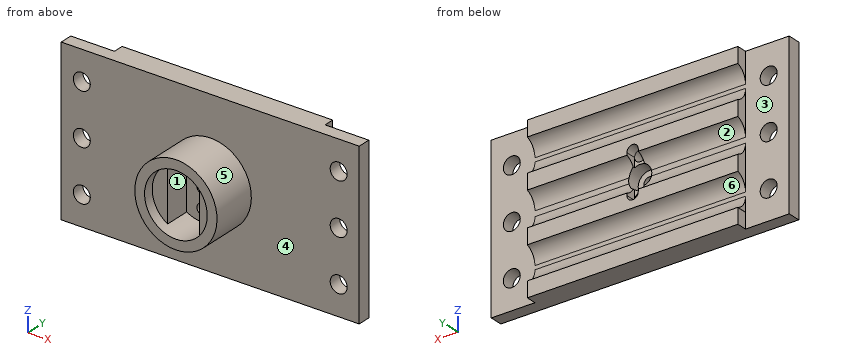
from build123d import *

# Parameters (mm, degrees)
SKETCH_1_R               = 50
EXTRUDE_1_DEPTH          = 2.5
SKETCH_2_R               = 8
EXTRUDE_2_DEPTH          = 9
SKETCH_3_R               = 6.1
CUT_EXTRUDE_1_DEPTH      = 2
CUT_EXTRUDE_2_DEPTH      = 5
SKETCH_7_R               = 1.15
CUT_EXTRUDE_4_DEPTH      = 4.5
SKETCH_8_R               = 2.25
CUT_EXTRUDE_5_DEPTH      = 2.5
CUT_EXTRUDE_6_DEPTH      = 72.281133549
CUT_EXTRUDE_6_DEPTH_BACK = 72.281133549
SKETCH_11_R              = 1.1
SKETCH_14_R              = 1.65
CUT_EXTRUDE_7_DEPTH      = 2.5
CUT_EXTRUDE_START        = -2.5
SKETCH_15_R              = 50
SKETCH_15_W              = 58
SKETCH_15_H              = 31.5
CUT_EXTRUDE_8_DEPTH      = 2.5
SKETCH_16_W              = 41
SKETCH_16_H              = 3
EXTRUDE_4_DEPTH          = 2
CUT_EXTRUDE_9_DEPTH      = 2
FILLET_3_R               = 3


with BuildPart() as part:
    # Эскиз1 → Бобышка-Вытянуть1 (new body)
    with BuildSketch(Plane(origin=(0, 0, 0), x_dir=(1, 0, 0), z_dir=(0, 1, 0))):
        with Locations(Location((0, 0, 0), (0, 0, 270))):
            Circle(SKETCH_1_R)
    extrude(amount=EXTRUDE_1_DEPTH)

    # Эскиз2 → Бобышка-Вытянуть2 (add)
    with BuildSketch(Plane.XZ):
        with Locations(Location((0, 0, 0), (0, 0, 270))):
            Circle(SKETCH_2_R)
    extrude(amount=EXTRUDE_2_DEPTH)

    # Эскиз3 → Вырез-Вытянуть1 (cut)
    with BuildSketch(Plane.XZ.offset(9)):
        with Locations(Location((0, 0, 0), (0, 0, 270))):
            Circle(SKETCH_3_R)
    extrude(amount=-CUT_EXTRUDE_1_DEPTH, mode=Mode.SUBTRACT)

    # Эскиз4 → Вырез-Вытянуть2 (cut)
    with BuildSketch(Plane.XZ.offset(7)):
        with BuildLine():
            Line((-3.1, 5.253570215), (-3.1, -5.253570215))
            ThreePointArc((-3.1, -5.253570215), (0, -6.1), (3.1, -5.253570215))
            Line((3.1, -5.253570215), (3.1, 5.253570215))
            ThreePointArc((3.1, 5.253570215), (0, 6.1), (-3.1, 5.253570215))
        make_face()
    extrude(amount=-CUT_EXTRUDE_2_DEPTH, mode=Mode.SUBTRACT)

    # Эскиз7 → Вырез-Вытянуть4 (cut)
    with BuildSketch(Plane(origin=(0, 2.5, 0), x_dir=(1, 0, 0), z_dir=(0, 1, 0))):
        with Locations(Location((0, 0, 0), (0, 0, 270))):
            Circle(SKETCH_7_R)
    extrude(amount=-CUT_EXTRUDE_4_DEPTH, mode=Mode.SUBTRACT)

    # Эскиз8 → Вырез-Вытянуть5 (cut)
    with BuildSketch(Plane(origin=(0, 2.5, 0), x_dir=(1, 0, 0), z_dir=(0, 1, 0))):
        with Locations(Location((0, 0, 0), (0, 0, 270))):
            Circle(SKETCH_8_R)
    extrude(amount=-CUT_EXTRUDE_5_DEPTH, mode=Mode.SUBTRACT)

    # Эскиз11 → Вырез-Вытянуть6 (cut, two sides: drawn at the far end of the back side and taken through both)
    with BuildSketch(Plane.XZ.offset(-CUT_EXTRUDE_6_DEPTH_BACK)):
        with Locations(Location((0, 3.8, 0), (0, 0, 270))):
            Circle(SKETCH_11_R)
        with Locations(Location((0, -3.8, 0), (0, 0, 90))):
            Circle(SKETCH_11_R)
    extrude(amount=CUT_EXTRUDE_6_DEPTH + CUT_EXTRUDE_6_DEPTH_BACK, mode=Mode.SUBTRACT)

    # Эскиз14 → Вырез-Вытянуть7 (cut)
    with BuildSketch(Plane(origin=(0, 2.5, 0), x_dir=(1, 0, 0), z_dir=(0, 1, 0))):
        with Locations(Location((-25, 0, 0), (0, 0, 270))):
            Circle(SKETCH_14_R)
        with Locations(Location((-25, 10, 0), (0, 0, 270))):
            Circle(SKETCH_14_R)
        with Locations(Location((-25, -10, 0), (0, 0, 270))):
            Circle(SKETCH_14_R)
        with Locations(Location((25, -10, 0), (0, 0, 270))):
            Circle(SKETCH_14_R)
        with Locations(Location((25, 0, 0), (0, 0, 270))):
            Circle(SKETCH_14_R)
        with Locations(Location((25, 10, 0), (0, 0, 270))):
            Circle(SKETCH_14_R)
    extrude(amount=-CUT_EXTRUDE_7_DEPTH, mode=Mode.SUBTRACT)

    # Эскиз15 → Вырез-Вытянуть8 (cut)
    with BuildSketch(Plane(origin=(0, 2.5, 0), x_dir=(1, 0, 0), z_dir=(0, 1, 0)).offset(CUT_EXTRUDE_START)):
        Circle(SKETCH_15_R)
        Rectangle(SKETCH_15_W, SKETCH_15_H, mode=Mode.SUBTRACT)
    extrude(amount=CUT_EXTRUDE_8_DEPTH, mode=Mode.SUBTRACT)

    # Эскиз16 → Бобышка-Вытянуть4 (add)
    with BuildSketch(Plane(origin=(0, 2.5, 0), x_dir=(1, 0, 0), z_dir=(0, 1, 0))):
        with Locations((0, 14.25)):
            Rectangle(SKETCH_16_W, SKETCH_16_H)
        with Locations((0, 4.85)):
            Rectangle(SKETCH_16_W, SKETCH_16_H)
        with Locations((0, -4.85)):
            Rectangle(SKETCH_16_W, SKETCH_16_H)
        with Locations((0, -14.25)):
            Rectangle(SKETCH_16_W, SKETCH_16_H)
    extrude(amount=EXTRUDE_4_DEPTH)

    # Эскиз17 → Вырез-Вытянуть9 (cut)
    with BuildSketch(Plane(origin=(0, 2.5, 0), x_dir=(1, 0, 0), z_dir=(0, 1, 0))):
        with BuildLine():
            Line((-1.1, 3.8), (-1.1, 2.7))
            Line((-1.1, 2.7), (1.1, 2.7))
            Line((1.1, 2.7), (1.1, 3.8))
            ThreePointArc((1.1, 3.8), (0, 4.9), (-1.1, 3.8))
        make_face()
        with BuildLine():
            Line((-1.1, -3.8), (-1.1, -2.7))
            Line((-1.1, -2.7), (1.1, -2.7))
            Line((1.1, -2.7), (1.1, -3.8))
            ThreePointArc((1.1, -3.8), (0, -4.9), (-1.1, -3.8))
        make_face()
    extrude(amount=CUT_EXTRUDE_9_DEPTH, mode=Mode.SUBTRACT)

    # Скругление3
    # the kernel refuses this fillet: 3 mm, written as the material it adds along each edge
    with BuildSketch(Plane(origin=(20.5, 2.5, 12.75), x_dir=(0, 0, -1), z_dir=(-1, 0, 0)), Plane(origin=(-20.5, 2.5, 6.35), x_dir=(0, 0, 1), z_dir=(1, 0, 0))) as fillet_3_piece_1:
        with BuildLine():
            CenterArc((2.828427125, -3), FILLET_3_R, 90, 70.528779366)
            Line((0, -2), (-0.056568542, -1.98))
            ThreePointArc((-0.056568542, -1.98), (-0.06, -1), (-0.06, 0))
            Line((-0.06, 0), (0, 0.06))
            Line((0, 0.06), (2.828427125, 0.06))
            Line((2.828427125, 0.06), (2.828427125, 0))
        make_face()
    extrude(amount=41)
    with BuildSketch(Plane(origin=(20.5, 2.5, 3.35), x_dir=(0, 0, -1), z_dir=(-1, 0, 0))) as fillet_3_piece_2_section:
        with BuildLine():
            CenterArc((2.828427125, -3), FILLET_3_R, 90, 70.528779366)
            Line((0, -2), (-0.056568542, -1.98))
            ThreePointArc((-0.056568542, -1.98), (-0.06, -1), (-0.06, 0))
            Line((-0.06, 0), (0, 0.06))
            Line((0, 0.06), (2.828427125, 0.06))
            Line((2.828427125, 0.06), (2.828427125, 0))
        make_face()
    fillet_3_piece_2 = extrude(amount=19.4, mode=Mode.PRIVATE)
    fillet_3_piece_2 = fillet_3_piece_2 - Plane(origin=(0, 3.015381172, 0), x_dir=(0, 0, 1), z_dir=(0, 1, 0)) * Cylinder(2.25, 51, mode=Mode.PRIVATE)
    add(fillet_3_piece_2)
    with BuildSketch(Plane(origin=(20.5, 2.5, 3.35), x_dir=(0, 0, -1), z_dir=(-1, 0, 0))) as fillet_3_piece_3_section:
        with BuildLine():
            CenterArc((2.828427125, -3), FILLET_3_R, 90, 70.528779366)
            Line((0, -2), (-0.056568542, -1.98))
            ThreePointArc((-0.056568542, -1.98), (-0.06, -1), (-0.06, 0))
            Line((-0.06, 0), (0, 0.06))
            Line((0, 0.06), (2.828427125, 0.06))
            Line((2.828427125, 0.06), (2.828427125, 0))
        make_face()
    fillet_3_piece_3 = extrude(amount=26.471067812, mode=Mode.PRIVATE)
    fillet_3_piece_3 = fillet_3_piece_3 - Plane(origin=(0, 3.020982336, 0), x_dir=(0, 0, 1), z_dir=(0, 1, 0)) * Cylinder(2.25, 65, mode=Mode.PRIVATE)
    fillet_3_piece_3 = split(fillet_3_piece_3, bisect_by=Plane(origin=(-1.1, 3.020982336, 2.69327095), z_dir=(-1, 0, 0)), keep=Keep.TOP, mode=Mode.PRIVATE)
    add(fillet_3_piece_3)
    with BuildSketch(Plane(origin=(5.971067812, 2.5, 3.35), x_dir=(0, 0, -1), z_dir=(-1, 0, 0))) as fillet_3_piece_4_section:
        with BuildLine():
            CenterArc((2.828427125, -3), FILLET_3_R, 90, 70.528779366)
            Line((0, -2), (-0.056568542, -1.98))
            ThreePointArc((-0.056568542, -1.98), (-0.06, -1), (-0.06, 0))
            Line((-0.06, 0), (0, 0.06))
            Line((0, 0.06), (2.828427125, 0.06))
            Line((2.828427125, 0.06), (2.828427125, 0))
        make_face()
    fillet_3_piece_4 = extrude(amount=26.471067812, mode=Mode.PRIVATE)
    fillet_3_piece_4 = fillet_3_piece_4 - Plane(origin=(0, 3.020982326, 0), x_dir=(0, 0, 1), z_dir=(0, 1, 0)) * Cylinder(2.25, 65, mode=Mode.PRIVATE)
    fillet_3_piece_4 = split(fillet_3_piece_4, bisect_by=Plane(origin=(1.1, 3.020982326, 2.69327092), z_dir=(1, 0, 0)), keep=Keep.TOP, mode=Mode.PRIVATE)
    add(fillet_3_piece_4)
    with BuildSketch(Plane(origin=(-1.1, 2.5, 3.35), x_dir=(0, 0, -1), z_dir=(-1, 0, 0))) as fillet_3_piece_5_section:
        with BuildLine():
            CenterArc((2.828427125, -3), FILLET_3_R, 90, 70.528779366)
            Line((0, -2), (-0.056568542, -1.98))
            ThreePointArc((-0.056568542, -1.98), (-0.06, -1), (-0.06, 0))
            Line((-0.06, 0), (0, 0.06))
            Line((0, 0.06), (2.828427125, 0.06))
            Line((2.828427125, 0.06), (2.828427125, 0))
        make_face()
    fillet_3_piece_5 = extrude(amount=19.4, mode=Mode.PRIVATE)
    fillet_3_piece_5 = fillet_3_piece_5 - Plane(origin=(0, 3.015381179, 0), x_dir=(0, 0, 1), z_dir=(0, 1, 0)) * Cylinder(2.25, 51, mode=Mode.PRIVATE)
    add(fillet_3_piece_5)
    with BuildSketch(Plane(origin=(5.971067812, 2.5, -3.35), x_dir=(0, 0, 1), z_dir=(-1, 0, 0))) as fillet_3_piece_6_section:
        with BuildLine():
            CenterArc((2.828427125, 3), FILLET_3_R, 199.471220634, 70.528779366)
            Line((0, 2), (-0.056568542, 1.98))
            ThreePointArc((-0.056568542, 1.98), (-0.06, 1), (-0.06, 0))
            Line((-0.06, 0), (0, -0.06))
            Line((0, -0.06), (2.828427125, -0.06))
            Line((2.828427125, -0.06), (2.828427125, 0))
        make_face()
    fillet_3_piece_6 = extrude(amount=26.471067812, mode=Mode.PRIVATE)
    fillet_3_piece_6 = fillet_3_piece_6 - Plane(origin=(0, 3.020982336, 0), x_dir=(0, 0, 1), z_dir=(0, 1, 0)) * Cylinder(2.25, 65, mode=Mode.PRIVATE)
    fillet_3_piece_6 = split(fillet_3_piece_6, bisect_by=Plane(origin=(1.1, 3.020982336, -2.69327095), z_dir=(1, 0, 0)), keep=Keep.TOP, mode=Mode.PRIVATE)
    add(fillet_3_piece_6)
    with BuildSketch(Plane(origin=(-1.1, 2.5, -3.35), x_dir=(0, 0, 1), z_dir=(-1, 0, 0))) as fillet_3_piece_7_section:
        with BuildLine():
            CenterArc((2.828427125, 3), FILLET_3_R, 199.471220634, 70.528779366)
            Line((0, 2), (-0.056568542, 1.98))
            ThreePointArc((-0.056568542, 1.98), (-0.06, 1), (-0.06, 0))
            Line((-0.06, 0), (0, -0.06))
            Line((0, -0.06), (2.828427125, -0.06))
            Line((2.828427125, -0.06), (2.828427125, 0))
        make_face()
    fillet_3_piece_7 = extrude(amount=19.4, mode=Mode.PRIVATE)
    fillet_3_piece_7 = fillet_3_piece_7 - Plane(origin=(0, 3.015381172, 0), x_dir=(0, 0, 1), z_dir=(0, 1, 0)) * Cylinder(2.25, 51, mode=Mode.PRIVATE)
    add(fillet_3_piece_7)
    with BuildSketch(Plane(origin=(20.5, 2.5, -3.35), x_dir=(0, 0, 1), z_dir=(-1, 0, 0))) as fillet_3_piece_8_section:
        with BuildLine():
            CenterArc((2.828427125, 3), FILLET_3_R, 199.471220634, 70.528779366)
            Line((0, 2), (-0.056568542, 1.98))
            ThreePointArc((-0.056568542, 1.98), (-0.06, 1), (-0.06, 0))
            Line((-0.06, 0), (0, -0.06))
            Line((0, -0.06), (2.828427125, -0.06))
            Line((2.828427125, -0.06), (2.828427125, 0))
        make_face()
    fillet_3_piece_8 = extrude(amount=19.4, mode=Mode.PRIVATE)
    fillet_3_piece_8 = fillet_3_piece_8 - Plane(origin=(0, 3.015381179, 0), x_dir=(0, 0, 1), z_dir=(0, 1, 0)) * Cylinder(2.25, 51, mode=Mode.PRIVATE)
    add(fillet_3_piece_8)
    with BuildSketch(Plane(origin=(20.5, 2.5, -3.35), x_dir=(0, 0, 1), z_dir=(-1, 0, 0))) as fillet_3_piece_9_section:
        with BuildLine():
            CenterArc((2.828427125, 3), FILLET_3_R, 199.471220634, 70.528779366)
            Line((0, 2), (-0.056568542, 1.98))
            ThreePointArc((-0.056568542, 1.98), (-0.06, 1), (-0.06, 0))
            Line((-0.06, 0), (0, -0.06))
            Line((0, -0.06), (2.828427125, -0.06))
            Line((2.828427125, -0.06), (2.828427125, 0))
        make_face()
    fillet_3_piece_9 = extrude(amount=26.471067812, mode=Mode.PRIVATE)
    fillet_3_piece_9 = fillet_3_piece_9 - Plane(origin=(0, 3.020982325, 0), x_dir=(0, 0, 1), z_dir=(0, 1, 0)) * Cylinder(2.25, 65, mode=Mode.PRIVATE)
    fillet_3_piece_9 = split(fillet_3_piece_9, bisect_by=Plane(origin=(-1.1, 3.020982325, -2.69327092), z_dir=(-1, 0, 0)), keep=Keep.TOP, mode=Mode.PRIVATE)
    add(fillet_3_piece_9)
    with BuildSketch(Plane(origin=(-20.5, 2.5, -6.35), x_dir=(0, 0, -1), z_dir=(1, 0, 0)), Plane(origin=(20.5, 2.5, -12.75), x_dir=(0, 0, 1), z_dir=(-1, 0, 0))) as fillet_3_piece_10:
        with BuildLine():
            CenterArc((2.828427125, 3), FILLET_3_R, 199.471220634, 70.528779366)
            Line((0, 2), (-0.056568542, 1.98))
            ThreePointArc((-0.056568542, 1.98), (-0.06, 1), (-0.06, 0))
            Line((-0.06, 0), (0, -0.06))
            Line((0, -0.06), (2.828427125, -0.06))
            Line((2.828427125, -0.06), (2.828427125, 0))
        make_face()
    extrude(amount=41)


solid = part.part
Read the model definition and answer for the solid it produces. Units are mm, in the model's axes. Face numbers are marked on the shaded views. A direction names the side the tool comes from. Give positions to 0.01 mm unless a question says otherwise; leave off trailing zeros. Write each loop counter-clockwise with the first axis right and the second up, starting at its lowest first coordinate (ties: lowest second). Pieces come first, ordered by that corner, then holes. Notation, with made-up numbers: (14, 47.25) - (30, 47.25) arc R15 ccw to (30, 52.25) - close; hole circle Ø3 at (57.5, 85.5). An arc over 180 degrees is marked (long way). Use CSV: the item, a comma, the result in double quotes. Start each with the question number.
Item 1: The part is cut by section B-B, the plane z = -11. Give the vertices of the cut face in (x, y).
Item 2: Consider line 1 (X direction, y = 1.5, z = 10); line 2 (X direction, y = 1.4, z = 0); line 3 (X direction, y = -5.25, z = 0). Determine where each line is inside the solid, lowest interval first.
Item 3: The part is cut by section A-A, the plane x = 25. Give the vertices of the cut face in (y, z).
Item 4: The part is cut by section D-D, the plane y = -1.25. Give the vertices of the cut face in (x, z), and give its area (3 significant figures).
Item 5: Flat-ended cylindrical pins translate along their axes: P1, Ø0.6, axis at y = 3.5, z = -5.5, coming from the -X side; P2, Ø5, axis at x = 0, z = 0.5, coming from the +Y side; P3, Ø3, axis at x = 0, z = -3.8, coming from the -Y side; P4, Ø8, axis at x = -17.5, y = -6.5, coming from the +Z side. Find the tip coordinate at first contact, or state that the pin passes through.
Item 6: The part is cut by section C-C, the plane y = -4.5. Give the vertices of the cut face in (x, z), and give its area (3 significant figures).
Item 7: The mould has two halves that part along Z. Classify the marked faces 4, 5 and 6: pulls with the +Z half, pulls with the -Z half, needs draft (parallel to the pull), parting line crosses it, or undercut.
Item 8: For the marked faces 1, 2 and 3, determine the directions among +Z, -Z, +X, -X, +Y, -Y from which every point of the face is accessible in a straight line to the end or side of a thin tool.
Taken from the geometry:
1,outline,"(-29, 0) - (-26.31, 0) - (-26.31, 2.5) - (-29, 2.5) - close; (-23.69, 0) - (23.69, 0) - (23.69, 2.5) - (20.5, 2.5) - (20.5, 2.7) - (-20.5, 2.7) - (-20.5, 2.5) - (-23.69, 2.5) - close; (26.31, 0) - (29, 0) - (29, 2.5) - (26.31, 2.5) - close"
2,line 1,"-29 to -26.65, -23.35 to 23.35, 26.65 to 29"
2,line 2,"-29 to -26.65, -23.35 to -2.25, 2.25 to 23.35, 26.65 to 29"
2,line 3,"-8 to -3.1, 3.1 to 8"
3,outline,"(0, -15.75) - (2.5, -15.75) - (2.5, -11.65) - (0, -11.65) - close; (0, -8.35) - (2.5, -8.35) - (2.5, -1.65) - (0, -1.65) - close; (0, 1.65) - (2.5, 1.65) - (2.5, 8.35) - (0, 8.35) - close; (0, 11.65) - (2.5, 11.65) - (2.5, 15.75) - (0, 15.75) - close"
4,outline,"circle Ø16 at (0, 0); hole circle Ø2.3 at (0, 0); hole circle Ø2.2 at (0, -3.8); hole circle Ø2.2 at (0, 3.8)"
4,area,"189 mm2"
5,P1,"x = -20.5"
5,P2,"y = 3.49"
5,P3,"y = -2"
5,P4,"through"
6,outline,"circle Ø16 at (0, 0); hole (-3.1, -5.25) arc R6.1 ccw to (3.1, -5.25) - (3.1, 5.25) arc R6.1 ccw to (-3.1, 5.25) - close"
6,area,"129 mm2"
7,face 4,"needs draft"
7,face 5,"parting line crosses it"
7,face 6,"undercut"
8,face 1,"-Y"
8,face 2,"+X, -X, +Y"
8,face 3,"+Y"
